from build123d import *

# Parameters (mm, degrees)
SKETCH004_W             = 105
SKETCH004_H             = 300
PAD004_DEPTH            = 5
SKETCH125_W             = 5
SKETCH125_H             = 10
POCKET035_DEPTH         = 5
LINEARPATTERN077_COUNT  = 15
LINEARPATTERN077_PITCH  = 20
SKETCH126_W             = 10
SKETCH126_H             = 5
POCKET036_DEPTH         = 5
LINEARPATTERN078_COUNT  = 5
LINEARPATTERN078_PITCH  = 20
BODY004_PLACEMENT_ANGLE = 90


with BuildPart() as part:
    # Sketch004 → Pad004 (new body)
    with BuildSketch(Plane.XY):
        Rectangle(SKETCH004_W, SKETCH004_H)
    extrude(amount=PAD004_DEPTH)

    # Sketch125 (on DatumPlane) → Pocket035 (cut)
    with BuildSketch(Plane.XY.offset(5)):
        with Locations((-50, 140)):
            Rectangle(SKETCH125_W, SKETCH125_H)
    pocket035 = extrude(amount=-POCKET035_DEPTH, mode=Mode.SUBTRACT)

    # LinearPattern077: Pocket035 ×15
    with Locations(*[(0, -i * LINEARPATTERN077_PITCH, 0) for i in range(1, LINEARPATTERN077_COUNT)]):
        add(pocket035, mode=Mode.SUBTRACT)

    # Sketch126 (on DatumPlane) → Pocket036 (cut)
    with BuildSketch(Plane.XY.offset(5)):
        with Locations((-37.5, 147.5)):
            Rectangle(SKETCH126_W, SKETCH126_H)
        with Locations((-37.5, -47.5)):
            Rectangle(SKETCH126_W, SKETCH126_H)
        with Locations((-37.5, -147.5)):
            Rectangle(SKETCH126_W, SKETCH126_H)
    pocket036 = extrude(amount=-POCKET036_DEPTH, mode=Mode.SUBTRACT)

    # LinearPattern078: Pocket036 ×5
    with Locations(*[(i * LINEARPATTERN078_PITCH, 0, 0) for i in range(1, LINEARPATTERN078_COUNT)]):
        add(pocket036, mode=Mode.SUBTRACT)


with BuildPart() as part_1:
    # Body004 placement: moved
    add(part.part.moved(Location((-250, 0, 52.5))).rotate(Axis((-250, 0, 52.5), (0, -1, 0)), BODY004_PLACEMENT_ANGLE))


solid = part_1.part
Can you work these out from the model? Positions are in its coordinate system, mm. A direction names the side the tool comes from. Coordinates: 2 decimals unless noted, no trailing zeros. Write each loop counter-clockwise with the first axis right and the second up, starting at its lowest first coordinate (ties: lowest second). Pieces come first, ordered by that corner, then holes. Notation, with made-up numbers: (71.5, 14) -> (94.5, 14) arc R29 ccw to (94.5, 53) -> close; hole circle Ø9 at (10.25, 5.25). An arc over 180 degrees is marked (long way). Answer as CSV lines item,"result".
1) If we section it at B-B on y = 79.5: Please give me the cut outline in (x, z).
Check result:
outline,"(-255, 5) -> (-250, 5) -> (-250, 105) -> (-255, 105) -> close"
2) If we section it at A-A on z = 93: Please give me the cut outline in (x, y).
Check result:
outline,"(-255, -145) -> (-250, -145) -> (-250, -50) -> (-255, -50) -> close; (-255, -45) -> (-250, -45) -> (-250, 145) -> (-255, 145) -> close"
3) Will these pins go through, and if not, where does the flat tip stop? P1, Ø2.5, axis at x = -252.5, y = 148.5, coming from the -Z side; P2, Ø2.5, axis at x = -251.5, z = 77.5, coming from the +Y side; P3, Ø2.5, axis at x = -253.5, y = -40, coming from the -Z side.
Check result:
P1,"z = 0"
P2,"y = 145"
P3,"z = 5"
4) On a 3-axis mill with a long thin cutter (end or side, diameter ignored), from which of +Z, -Z, +X, -X, +Y, -Y can I reach the whole of each face in a straight line? I mean faces 1 (the flat face through (-253, 20, 5)), 2 (the flat face through (-253, -50, 55)), 3 (the flat face through (-253, 145, 55)), 4 (the flat face through (-253, -145, 55)), 5 (the flat face through (-252, -2, 105)). Say none if no direction works.
Check result:
face 1,"-Z, +X, -X"
face 2,"+X, -X"
face 3,"+X, -X, +Y"
face 4,"+X, -X, -Y"
face 5,"+Z, +X, -X, +Y, -Y"
5) If we section it at C-C on x = -252.65: Count the separate pieces of the cut face and the enclosed holes in it, then the cut area to 3 significant figures.
Check result:
separate pieces,"1"
enclosed holes,"5"
area,"30,000 mm²"
6) If we mould it in two halves opening along Z, with no side actions, what happens to faces 6 (the flat face through (-252, -150, 45)), 7 (the flat face through (-253, -148, 60)), 8 (the flat face through (-252, -130, 0)), 9 (the flat face through (-253, 147, 80))? For each: +Z half, -Z half, draft (parallel to the pull), parting line (faces both ways), or undercut.
Check result:
face 6,"draft"
face 7,"undercut"
face 8,"-Z half"
face 9,"undercut"
7) If I drill on line 1 (Y direction, x = -250.35, z = 54.5); line 2 (Z direction, x = -254.1, y = -2.5), over which ranges is the centre line in solid material (lowest first)? Write a range as from..to.
Check result:
line 1,"-145..-50, -45..145"
line 2,"5..105"
